Check sheet for the modelled part. Datum: model origin and axes. Units: mm. A direction names the side the tool comes from. Coordinates: 2 decimals unless noted, no trailing zeros. Write each loop counter-clockwise with the first axis right and the second up, starting at its lowest first coordinate (ties: lowest second). Pieces come first, ordered by that corner, then holes. Notation, with made-up numbers: M 8,36 L 23,36 A16 ccw 23,46 Z; hole C -30,45.25 d11. An arc over 180 degrees is marked long. Answer as CSV lines item,"result".
Autodesk Inventor part; units mm, degrees
ref_plane "YZ Plane" through (0, 0, 0) normal (1, 0, 0) x (0, 1, 0)
ref_plane "XZ Plane" through (0, 0, 0) normal (0, 1, 0) x (-1, 0, 0)
ref_plane "XY Plane" through (0, 0, 0) normal (0, 0, 1) x (1, 0, 0)
sketch "Sketch1" plane through (0, 0, 0) normal (0, 1, 0) x (-1, 0, 0)
  line L0 (-54.2742, 0) -> (84.3226, 0) construction
  line L1 (-6.35, -36.068) -> (69.85, -36.068)
  line L2 (69.85, -36.068) -> (69.85, 36.068)
  line L3 (69.85, 36.068) -> (-6.35, 36.068)
  line L4 (-31.75, 10.668) -> (-31.75, -10.668)
  circle A0 centre (0, 0) radius 17 construction
  circle A1 centre (0, 0) radius 20.81
  line L5 (0, 0) -> (-18.9066, 32.7472) construction
  circle A2 centre (0, 0) radius 3.81 construction
  arc A3 (-6.35, 36.068) -> (-31.75, 10.668) centre (-6.35, 10.668) ccw
  arc A4 (-31.75, -10.668) -> (-6.35, -36.068) centre (-6.35, -10.668) ccw
  circle A5 centre (-12.2465, 21.2116) radius 1.6256
  line L6 (0, 0) -> (31.1733, 53.9938) construction
  circle A6 centre (24.493, 0) radius 1.6256
  circle A7 centre (-12.2465, -21.2116) radius 1.6256
  circle A8 centre (-12.2465, 21.2116) radius 3.175 construction
  line L7 (-57.1489, 10.668) -> (-67.0521, 10.668)
  line L8 (-67.0521, 10.668) -> (-67.0521, -7.3902)
  line L9 (-67.0521, -7.3902) -> (-57.1489, -7.3902)
  line L10 (-57.1489, -7.3902) -> (-57.1489, 10.668)
  point P0 (-31.75, -36.068)
  point P1 (-31.75, 36.068)
  dimension "d0" = 72.136
  dimension "d1" = 101.6
  dimension "d2" = 34
  dimension "d3" = 3.81
  dimension "d4" = 31.75
  dimension "tri_angle" = 120
  dimension "fov_diameter" = 7.62
  dimension "d9" = 25.4
  dimension "d12" = 3.2512
  dimension "mount_radius" = 24.493
  dimension "d14" = 60
  dimension "d25" = 6.35
  dimension "main_aperture_diameter" = 41.62
  dimension "d67" = 2.0574
  dimension "d68" = 10.94
extrude "Extrusion2" add sketch "Sketch1" against normal blind 12.7 contours A4 L4 A3 L3 L2 L1
sketch "Sketch2" plane through (0, -12.7, 0) normal (0, -1, 0) x (1, 0, 0)
  line L0 (0, 0) -> (-53.7265, 0) construction
  circle A0 centre (0, 0) radius 20.81
  circle A1 centre (12.2465, -21.2116) radius 1.6256
  circle A2 centre (-24.493, 0) radius 1.6256
  circle A3 centre (12.2465, 21.2116) radius 1.6256
  line L1 (-69.85, 36.068) -> (-69.85, -36.068)
  line L2 (6.35, 36.068) -> (-69.85, 36.068)
  arc A4 (31.75, 10.668) -> (6.35, 36.068) centre (6.35, 10.668) ccw
  line L3 (31.75, -10.668) -> (31.75, 10.668)
  arc A5 (6.35, -36.068) -> (31.75, -10.668) centre (6.35, -10.668) ccw
  line L4 (-69.85, -36.068) -> (6.35, -36.068)
  line L5 (54.2742, 0) -> (-84.3226, 0) construction
  line L6 (0, 0) -> (-31.1733, 53.9938) construction
  circle A6 centre (0, 0) radius 17 construction
  circle A7 centre (0, 0) radius 3.81 construction
  line L7 (0, 0) -> (18.9066, 32.7472) construction
  line L8 (41.6502, 64.7743) -> (11.4877, 12.5313) construction
  line L9 (11.4877, 12.5313) -> (41.6502, 64.7743) construction
  line L10 (10.1129, 13.325) -> (40.2754, 65.568)
  line L11 (43.025, 63.9805) -> (12.8625, 11.7375)
  arc A8 (10.1129, 13.325) -> (12.8625, 11.7375) centre (11.4877, 12.5313) ccw
  arc A9 (43.025, 63.9805) -> (40.2754, 65.568) centre (41.6502, 64.7743) ccw
  line L12 (6.4834, 15.4205) -> (36.6459, 67.6635)
  line L13 (33.8962, 69.251) -> (3.7337, 17.008)
  arc A10 (3.7337, 17.008) -> (6.4834, 15.4205) centre (5.1086, 16.2143) ccw
  arc A11 (36.6459, 67.6635) -> (33.8962, 69.251) centre (35.2711, 68.4573) ccw
  line L14 (10.1129, -13.325) -> (40.2754, -65.568)
  line L15 (43.025, -63.9805) -> (12.8625, -11.7375)
  arc A12 (12.8625, -11.7375) -> (10.1129, -13.325) centre (11.4877, -12.5313) ccw
  arc A13 (40.2754, -65.568) -> (43.025, -63.9805) centre (41.6502, -64.7743) ccw
  arc A14 (33.8962, -69.251) -> (36.6459, -67.6635) centre (35.2711, -68.4573) ccw
  line L16 (33.8962, -69.251) -> (3.7337, -17.008)
  arc A15 (6.4834, -15.4205) -> (3.7337, -17.008) centre (5.1086, -16.2143) ccw
  line L17 (6.4834, -15.4205) -> (36.6459, -67.6635)
  line L18 (-16.5962, -2.0955) -> (-76.9212, -2.0955)
  line L19 (-76.9212, -5.2705) -> (-16.5962, -5.2705)
  arc A16 (-16.5962, -5.2705) -> (-16.5962, -2.0955) centre (-16.5962, -3.683) ccw
  arc A17 (-76.9212, -2.0955) -> (-76.9212, -5.2705) centre (-76.9212, -3.683) ccw
  arc A18 (-76.9212, 5.2705) -> (-76.9212, 2.0955) centre (-76.9212, 3.683) ccw
  line L20 (-76.9212, 5.2705) -> (-16.5962, 5.2705)
  arc A19 (-16.5962, 2.0955) -> (-16.5962, 5.2705) centre (-16.5962, 3.683) ccw
  line L21 (-16.5962, 2.0955) -> (-76.9212, 2.0955)
  point P0 (26.5689, 38.6528)
  dimension "d20" = 3.683
  dimension "pin_diameter" = 3.175
  dimension "d28" = 63.5
extrude "Extrusion3" cut sketch "Sketch2" against normal blind 2.921 contours L11 A8 L10 A0 | A0 L10 A4 L11 | L15 A5 L14 A0 | A0 L14 A12 L15 | A4 L10 A9 L11 | L15 A13 L14 A5 | L12 A10 L13 A0 | A0 L13 A4 L12 | L17 A5 L16 A0 | A0 L16 A15 L17 | A4 L13 A11 L12 | L17 A14 L16 A5 | L20 A19 L21 A0 | A0 L21 L1 L20 | L19 L1 L18 A0 | A0 L18 A16 L19 | L1 L21 A18 L20 | L19 A17 L18 L1
sketch "Sketch3" plane through (0, 0, 0) normal (0, 1, 0) x (1, 0, 0)
  circle A0 centre (12.2465, -21.2116) radius 3.175 construction
  circle A1 centre (12.2465, -21.2116) radius 3.175
  line L0 (54.2742, 0) -> (-84.3226, 0) construction
  line L1 (0, 0) -> (-31.1733, -53.9938) construction
  circle A2 centre (12.2465, 21.2116) radius 3.175
  circle A3 centre (-24.493, 0) radius 3.175
extrude "Extrusion4" cut sketch "Sketch3" against normal blind 9.779
sketch "Sketch4" plane through (0, 0, 0) normal (0, 1, 0) x (1, 0, 0)
  line L0 (54.2742, 0) -> (-84.3226, 0) construction
  line L1 (-63.5, -29.1592) -> (-12.7, -29.1592) construction
  line L2 (-63.5, -26.67) -> (-12.7, -26.67)
  line L3 (-12.7, -31.6484) -> (-63.5, -31.6484)
  arc A0 (-63.5, -26.67) -> (-63.5, -31.6484) centre (-63.5, -29.1592) ccw
  arc A1 (-12.7, -31.6484) -> (-12.7, -26.67) centre (-12.7, -29.1592) ccw
  line L4 (-63.5, 26.67) -> (-12.7, 26.67)
  line L5 (-12.7, 31.6484) -> (-63.5, 31.6484)
  arc A2 (-63.5, 31.6484) -> (-63.5, 26.67) centre (-63.5, 29.1592) ccw
  arc A3 (-12.7, 26.67) -> (-12.7, 31.6484) centre (-12.7, 29.1592) ccw
  point P0 (0, 0)
  point P1 (-38.1, -29.1592)
  dimension "d33" = 4.9784
  dimension "d34" = 50.8
  dimension "d35" = 58.3184
  dimension "d36" = 12.7
sketch "Sketch5" plane through (0, -12.7, 0) normal (0, -1, 0) x (1, 0, 0)
  circle A0 centre (12.2465, 21.2116) radius 1.6256
  line L0 (0, 0) -> (18.9066, 32.7472) construction
  line L1 (54.2742, 0) -> (-84.3226, 0) construction
  line L2 (0, 0) -> (-31.1733, 53.9938) construction
  circle A1 centre (12.2465, 21.2116) radius 3.175 construction
  line L3 (9.4969, 22.7991) -> (6.9569, 18.3997)
  line L4 (14.9961, 19.6241) -> (12.4561, 15.2247)
  line L5 (6.9569, 18.3997) -> (12.4561, 15.2247)
  arc A2 (14.9961, 19.6241) -> (9.4969, 22.7991) centre (12.2465, 21.2116) ccw
  line L6 (-24.493, 3.175) -> (-19.413, 3.175)
  line L7 (-24.493, -3.175) -> (-19.413, -3.175)
  line L8 (-19.413, 3.175) -> (-19.413, -3.175)
  arc A3 (-24.493, 3.175) -> (-24.493, -3.175) centre (-24.493, 0) ccw
  line L9 (9.4969, -22.7991) -> (6.9569, -18.3997)
  line L10 (14.9961, -19.6241) -> (12.4561, -15.2247)
  line L11 (6.9569, -18.3997) -> (12.4561, -15.2247)
  arc A4 (9.4969, -22.7991) -> (14.9961, -19.6241) centre (12.2465, -21.2116) ccw
  dimension "d50" = 5.08
extrude "Extrusion6" [suppressed]
extrude "Extrusion7" [suppressed]
sketch "Sketch6" plane through (0, 0, 0) normal (0, 1, 0) x (1, 0, 0)
  line L0 (0, 0) -> (18.9066, -32.7472) construction
  line L1 (41.6502, -64.7743) -> (11.4877, -12.5313) construction
  line L2 (0, 0) -> (33.579, -42.2146) construction
  circle A0 centre (15.5113, -19.5004) radius 3.175
  circle A1 centre (9.1322, -23.1834) radius 3.175
  line L3 (0, 0) -> (-31.1733, -53.9938) construction
  line L4 (54.2742, 0) -> (-84.3226, 0) construction
  circle A2 centre (-24.6435, 3.683) radius 3.175
  circle A3 centre (-24.6435, -3.683) radius 3.175
  circle A4 centre (15.5113, 19.5004) radius 3.175
  circle A5 centre (9.1322, 23.1834) radius 3.175
  dimension "d45" = 8.5
  dimension "d46" = 6.35
extrude "Extrusion8" [suppressed]
chamfer "Chamfer2" [suppressed]
sketch "Sketch7" plane through (0, -12.7, 0) normal (0, -1, 0) x (1, 0, 0)
  line L0 (0, 0) -> (-31.1733, 53.9938) construction
  line L1 (0, 0) -> (18.9066, 32.7472) construction
  circle A0 centre (12.2465, 21.2116) radius 3.175
  circle A1 centre (-24.493, 0) radius 3.175
  line L2 (54.2742, 0) -> (-84.3226, 0) construction
  circle A2 centre (12.2465, -21.2116) radius 3.175
  dimension "d54" = 6.35
extrude "Extrusion9" cut sketch "Sketch7" against normal blind 2.159
sketch "Sketch8" plane through (0, 0, 0) normal (0, 1, 0) x (1, 0, 0)
  circle A0 centre (0, 0) radius 20.81
  line L0 (54.2742, 0) -> (-84.3226, 0) construction
  line L1 (0, 0) -> (12.8396, -66.0541) construction
  point P0 (4.3134, -22.1907)
  point P1 (4.3134, 22.1907)
  dimension "d57" = 101
  dimension "d58" = 22.606
hole "Hole1" at (4.3134, 0, 22.1907) at (4.3134, 0, -22.1907) direction (0, -1, 0) diameter 1.27 depth 25.4 tip angle 118
sketch "Sketch9" plane through (0, 0, 0) normal (0, 1, 0) x (1, 0, 0)
  line L0 (0, 0) -> (22.9874, -39.8154) construction
  line L1 (15.2539, -22.2295) -> (20.6849, -31.6363)
  circle A0 centre (12.2465, -21.2116) radius 3.175
  line L2 (12.2465, -21.2116) -> (22.1452, -15.4966) construction
  point P0 (17.1958, -18.3541)
  point P1 (7.2972, -24.0691)
  dimension "d69" = 11.43
hole "Hole2" at (17.1958, 0, 18.3541) at (7.2972, 0, 24.0691) direction (0, -1, 0) diameter 1.7018 depth 12.7 tip angle 118
sketch "Sketch10" plane through (0, 0, 0) normal (0, 1, 0) x (1, 0, 0)
  circle A0 centre (-24.493, 0) radius 3.175
  line L0 (0, 50.4952) -> (0, -50.4952)
  line L1 (0, 0) -> (18.9066, -32.7472) construction
  circle A1 centre (24.493, 0) radius 3.175
  line L2 (0, 0) -> (37.8406, -21.8473) construction
  point P0 (7.2972, -24.0691)
  point P1 (17.1958, -18.3541)
  point P2 (24.493, 5.715)
  point P3 (24.493, -5.715)
  dimension "d77" = 30
extrude "Extrusion10" cut sketch "Sketch10" against normal blind 25.4 contours A1
sketch "Sketch11" plane through (0, 0, 0) normal (0, 1, 0) x (1, 0, 0)
  point P0 (0, 0)
  point P1 (24.493, -5.715)
  point P2 (24.493, 5.715)
hole "Hole3" at (24.493, 0, 5.715) at (24.493, 0, -5.715) direction (0, -1, 0) diameter 1.7018 depth 12.7 tip angle 118
equation "\"fov_diameter\" = 2 * d3"
equation "\"d14\" = 0.5 * tri_angle"
equation "\"d15\" = plate_thickness"
equation "\"d23\" = pin_depth"
equation "\"d26\" = magnet_depth"
equation "\"d40\" = bearing_relief_depth"
equation "\"d46\" = magnet_diameter"
equation "\"d47\" = magnet_depth"
equation "\"d54\" = magnet_diameter"
equation "\"d55\" = bearing_relief_depth"
equation "\"plate_thickness\" = 12.7"
equation "\"magnet_depth\" = plate_thickness - pin_depth"
equation "\"hole_diameter\" = d2 + fov_diameter"
properties part number "tri_mount"
1) Section check D-D, the plane x = -47.5. Record the boundary of the cut face in (y, z), plus the area to 3 significant figures.
Answer key:
outline,"M -12.7,-36.07 L 0,-36.07 L 0,36.07 L -12.7,36.07 L -12.7,5.27 L -9.78,5.27 L -9.78,2.1 L -12.7,2.1 L -12.7,-2.1 L -9.78,-2.1 L -9.78,-5.27 L -12.7,-5.27 Z"
area,"898 mm2"
2) Thickness scan on line 1 along X through (y, z) = (-8.25, 0); line 2 along X through (y, z) = (-1.5, -0.5); line 3 along Z through (x, y) = (10.5, -6.75). Record the ranges inside material, lowest first.
Answer key:
line 1,"x = -69.85 to -27.67, -21.32 to -20.81, 20.81 to 21.32, 27.67 to 31.75"
line 2,"x = -69.85 to -27.63, -21.36 to -20.8, 20.8 to 21.36, 27.63 to 31.75"
line 3,"z = -35.73 to -23.86, -18.56 to -17.97, 17.97 to 18.56, 23.86 to 35.73"
3) Section check C-C, the plane y = -2.5. Give the number of separate pieces and of enclosed holes in the cut face, plus the area to 3 significant figures.
Answer key:
separate pieces,"1"
enclosed holes,"11"
area,"5,550 mm2"
4) Section check B-B, the plane x = 0. Record the boundary of the cut face in (y, z), plus the area to 3 significant figures.
Answer key:
outline,"M -12.7,-36.07 L 0,-36.07 L 0,-20.81 L -12.7,-20.81 Z; M -12.7,20.81 L 0,20.81 L 0,36.07 L -12.7,36.07 Z"
area,"388 mm2"
5) Mould release check, pull along Z, two halves, no side actions. Record for faces 1 (the face through (-32, -6, 36.068)), 2 (the face through (13.5, -10.541, 19.8)), 3 (the face through (-27.668, -11.636, 0.032)), 4 (the face through (31.75, -6, 0)): pulls with the +Z half, pulls with the -Z half, needs draft (parallel to the pull), parting line crosses it, or undercut.
Answer key:
face 1,"pulls with the +Z half"
face 2,"undercut"
face 3,"undercut"
face 4,"needs draft"
6) Tool access check on faces 5 (the face through (16, -12.7, -28)), 6 (the face through (15.275, -4.821, 20.258)), 7 (the face through (-23, -10.541, 1)). Record the directions out of +Z, -Z, +X, -X, +Y, -Y that give a thin tool (end or side, any length) a straight path to the whole face; none if there is none.
Answer key:
face 5,"+Z, -Z, +X, -X, -Y"
face 6,"+Y"
face 7,"-Y"
7) Section check A-A, the plane z = 0. Record the boundary of the cut face in (x, y).
Answer key:
outline,"M -69.85,-12.7 L -27.67,-12.7 L -27.67,-10.54 L -26.12,-10.54 L -26.12,-9.78 L -27.67,-9.78 L -27.67,0 L -69.85,0 Z; M -22.87,-10.54 L -21.32,-10.54 L -21.32,-12.7 L -20.81,-12.7 L -20.81,0 L -21.32,0 L -21.32,-9.78 L -22.87,-9.78 Z; M 20.81,-12.7 L 21.32,-12.7 L 21.32,0 L 20.81,0 Z; M 27.67,-12.7 L 31.75,-12.7 L 31.75,0 L 27.67,0 Z"
8) Depth check by flat-ended pin: P1, Ø3, axis at x = 11, z = -21.5, coming from the +Y side; P2, Ø1.5, axis at x = 14, y = -10.5, coming from the -Z side; P3, Ø4.5, axis at x = -24.5, z = 0.5, coming from the -Y side. Enter the tip coordinate at first touch or a pass-through.
Answer key:
P1,"stops at y = -9.78"
P2,"stops at z = -35.11"
P3,"stops at y = -10.54"
